Input: part model. Units: mm. Frame: model coordinates. A direction names the side the tool comes from. Round coordinates to 2 decimals unless told otherwise and drop trailing zeros. Loops run counter-clockwise (first coordinate to the right, second up) from the corner with the lowest first, then second, coordinate; pieces in that order, holes last. Notation, with made-up numbers: M -2,14.25 L 36,14.25 A17 cw 36,45.25 Z; hole C -1.75,-39 d10. An arc over 180 degrees is marked long. Use one line per item in the form item = value. Start each with the question number.
Q1. Section query A-A, the plane x = 0. Output: boundary loops of the cut face in (y, z), and give its area (3 significant figures).
Q2. First-contact query: P1, Ø6, axis at y = 16.5, z = 6.5, coming from the +X side; P2, Ø0.8, axis at x = -21.5, z = 3, coming from the +Y side; P3, Ø0.8, axis at x = -22, z = 4.5, coming from the -Y side. Flat tips, straight axial feed; report the tip coordinate or a pass-through.
Q3. Access query for faces 4 (the cylindrical face through (-19.76, -13.06, 3.7)), 5 (the flat face through (1, 0, 10)). Directions: +Z, -Z, +X, -X, +Y, -Y. A direction counts if a zero-diameter tool reaches every point of the face in a straight line with its end or side. Return the directions, or none.
Q4. Ray query, line 1 along Y through (x, z) = (0, 4); line 2 along Z through (x, y) = (3, 20); line 3 along X through (y, z) = (0, 4). Return the intervals inside material, ascending.
Q5. Section query C-C, the plane z = 5.25. Output: boundary loops of the cut face in (x, y).
Q6. Section query B-B, the plane y = 0. Output: boundary loops of the cut face in (x, z).
Q7. Mould query, pull axis X, two halves, no side actions, for faces 1 (the flat face through (-17.3, 15.8, 0)), 2 (the flat face through (-22.25, 0, 9)), 3 (the cylindrical face through (-19.72, 13.08, 3.7)). Classes: pulls with the +X half, pulls with the -X half, needs draft (parallel to the pull), parting line crosses it, or undercut.
```python
from build123d import *

# Parameters (mm, degrees)
SKETCH_1_R          = 25.6
EXTRUDE_1_DEPTH     = 10
CHAMFER_1_SIZE      = 2
CUT_EXTRUDE_START   = -2.5
CUT_EXTRUDE_1_DEPTH = 2.5
SKETCH_3_R          = 23.2
CUT_EXTRUDE_2_DEPTH = 7.5
CUT_EXTRUDE_3_REACH = 39.56
SKETCH_5_W          = 9.365653714
SKETCH_5_H          = 25.321729798
FILLET_2_R          = 4


with BuildPart() as part:
    # Эскиз1 → Бобышка-Вытянуть1 (new body)
    with BuildSketch(Plane.XY):
        Circle(SKETCH_1_R)
    extrude(amount=EXTRUDE_1_DEPTH)

    # Фаска1
    chamfer_1_edges = [part.edges().sort_by_distance(p)[0] for p in [
        (-25.6, 0, 0),
    ]]
    chamfer(chamfer_1_edges, length=CHAMFER_1_SIZE)

    # Эскиз2 → Вырез-Вытянуть1 (cut)
    with BuildSketch(Plane.XY.offset(10).offset(CUT_EXTRUDE_START)):
        with BuildLine():
            Line((-22.25, -12.660864899), (-22.25, 12.660864899))
            ThreePointArc((-22.25, 12.660864899), (-25.6, 0), (-22.25, -12.660864899))
        make_face()
    extrude(amount=CUT_EXTRUDE_1_DEPTH, mode=Mode.SUBTRACT)

    # Эскиз3 → Вырез-Вытянуть2 (cut)
    with BuildSketch(Plane(origin=(0, 0, 0), x_dir=(-1, 0, 0), z_dir=(0, 0, -1))):
        Circle(SKETCH_3_R)
    extrude(amount=-CUT_EXTRUDE_2_DEPTH, mode=Mode.SUBTRACT)

    # Вырез-Вытянуть3: up to this face of the body (flat: up to its plane)
    cut_extrude_3_end = Plane(part.part.faces().sort_by_distance((0.112414177, 0, 7.5))[0])
    # Эскиз5 → Вырез-Вытянуть3 (cut, up to the picked face)
    with BuildSketch(Plane(origin=(0, 0, 0), x_dir=(-1, 0, 0), z_dir=(0, 0, -1)), mode=Mode.PRIVATE) as cut_extrude_3_sk1:
        with Locations((22.25, 0)):
            Rectangle(SKETCH_5_W, SKETCH_5_H)
    cut_extrude_3_tool1 = split(extrude(cut_extrude_3_sk1.sketch, amount=-CUT_EXTRUDE_3_REACH, mode=Mode.PRIVATE), bisect_by=cut_extrude_3_end, keep=Keep.BOTH, mode=Mode.PRIVATE)
    add(cut_extrude_3_tool1.solids().sort_by(Axis((-22.25, 0, 0), (0, 0, 1)))[0], mode=Mode.SUBTRACT)

    # Скругление2
    fillet_2_edges = [part.edges().sort_by_distance(p)[0] for p in [
        (-19.440743299, 12.660864899, 3.75),
        (-19.440743299, -12.660864899, 3.75),
    ]]
    fillet(fillet_2_edges, radius=FILLET_2_R)


solid = part.part
```
Results found:
q1.outline = M -25.6,2 L -23.6,0 L -23.2,0 L -23.2,7.5 L 23.2,7.5 L 23.2,0 L 23.6,0 L 25.6,2 L 25.6,10 L -25.6,10 Z
q1.area = 160 mm²
q2.P1 = 21.75
q2.P2 = 14.5
q2.P3 = -13.74
q3.face_4 = -Z
q3.face_5 = +Z, +X, -X, +Y, -Y
q4.line_1 = -25.6 to -23.2, 23.2 to 25.6
q4.line_2 = 7.5 to 10
q4.line_3 = 23.2 to 25.6
q5.outline = M -22.25,-12.66 A25.6 ccw long -22.25,12.66 L -21.5,12.66 A4 ccw -18.34,14.21 A23.2 cw long -18.34,-14.21 A4 ccw -21.5,-12.66 Z
q6.outline = M -22.25,7.5 L 23.2,7.5 L 23.2,0 L 23.6,0 L 25.6,2 L 25.6,10 L -22.25,10 Z
q7.face_1 = needs draft
q7.face_2 = pulls with the -X half
q7.face_3 = undercut
